```python
from build123d import *

# Parameters (mm, degrees)
SKETCH1_W           = 105
SKETCH1_H           = 100
BOSS_EXTRUDE1_DEPTH = 10
SKETCH4_R           = 15
BOSS_EXTRUDE2_DEPTH = 30
SKETCH5_R           = 4
CUT_EXTRUDE3_DEPTH  = 30
SKETCH6_W           = 42
SKETCH6_H           = 42
BOSS_EXTRUDE3_DEPTH = 1
SKETCH2_R           = 2.25
CUT_EXTRUDE4_DEPTH  = 99.994949366
BOSS_EXTRUDE4_START = 1
LOCAL_FILES1_R      = 6
LOCAL_FILES1_R_2    = 4
BOSS_EXTRUDE4_DEPTH = 1


with BuildPart() as part:
    # Sketch1 → Boss-Extrude1 (new body)
    with BuildSketch(Plane.XY):
        with Locations((-27.5, 0)):
            Rectangle(SKETCH1_W, SKETCH1_H)
    extrude(amount=BOSS_EXTRUDE1_DEPTH)

    # Sketch4 → Boss-Extrude2 (add)
    with BuildSketch(Plane.XY.offset(10)):
        Circle(SKETCH4_R)
    extrude(amount=BOSS_EXTRUDE2_DEPTH)

    # Sketch5 → Cut-Extrude3 (cut)
    with BuildSketch(Plane.XY.offset(40)):
        Circle(SKETCH5_R)
    extrude(amount=-CUT_EXTRUDE3_DEPTH, mode=Mode.SUBTRACT)

    # Sketch6 → Boss-Extrude3 (add)
    with BuildSketch(Plane.XY.offset(10)):
        with Locations((-59, 2.474517647)):
            Rectangle(SKETCH6_W, SKETCH6_H)
    extrude(amount=BOSS_EXTRUDE3_DEPTH)

    # Sketch2 → Cut-Extrude4 (cut, through all)
    with BuildSketch(Plane.XY.offset(10)):
        with Locations((-70, 40)):
            Circle(SKETCH2_R)
        with Locations((15, -40)):
            Circle(SKETCH2_R)
        with Locations(Location((-70, -40, 0), (0, 0, 180))):
            Circle(SKETCH2_R)
        with Locations(Location((15, 40, 0), (0, 0, 180))):
            Circle(SKETCH2_R)
    extrude(amount=-CUT_EXTRUDE4_DEPTH, mode=Mode.SUBTRACT)

    # Local Files1 → Boss-Extrude4 (add)
    with BuildSketch(Plane.XY.offset(40).offset(BOSS_EXTRUDE4_START)):
        Circle(LOCAL_FILES1_R)
        Circle(LOCAL_FILES1_R_2, mode=Mode.SUBTRACT)
    extrude(amount=-BOSS_EXTRUDE4_DEPTH)


solid = part.part
```
Here's how the part is built. I have some questions about the finished solid (model axes, mm). A direction names the side the tool comes from. Coordinates: 2 decimals unless noted, no trailing zeros. Order: outer loops, then holes, each group sorted by start corner. A loop starts at its lowest first (then second) coordinate and runs counter-clockwise, first axis right, second up. Notation, with made-up numbers: M 48.25,62 L 91.25,62 A17 cw 91.25,77 Z; hole C 39.5,-39 d3. An arc over 180 degrees is marked long. Answer as a JSON object with one key per item and string values. Group by question number.
(1) Suppose I cut it at A-A, the plane x = -65.5. Please give me the cut outline in (y, z).
(2) Suppose I cut it at C-C, the plane y = 40. Please give me the cut outline in (x, z), then the cut area to 3 significant figures.
(3) For pin 1 (0.8 mm diameter, centred on x = -53, z = 10.5, fed in from +Y); pin 2 (10 mm diameter, centred on x = 0, z = 24.5, fed in from -Y); pin 3 (1 mm diameter, centred on y = -10.5, z = 13, fed in from -X), each with a flat end and sliding along its axis, tell me the tip position at first contact or that it passes through.
(4) Suppose I cut it at B-B, the plane y = 0. Please give me the cut outline in (x, z), then the cut area to 3 significant figures.
(5) Which directions (+Z, -Z, +X, -X, +Y, -Y) give clear straight access to the entire face, cutting with the end or side of a thin tool? Please do faces 4 (the face through (-5.994, 0.264, 40.507)), 5 (the face through (-80, -1, 5)), 6 (the face through (-59, 3, 11)).
(6) If we mould it in two halves opening along X, with no side actions, what happens to faces 1 (the face through (25, -1, 5)), 2 (the face through (-1.42, -3.92, 41)), 3 (the face through (16.21, -38.103, 5.07))? For each: released by +X, released by -X, zero draft, split by the parting line, or undercut.
(7) Suppose I cut it at D-D, the plane z = 15.5. Please give me the cut outline in (x, y), then the cut area to 3 significant figures.
(8) I need wall thicknesses on probe 1 along Y at (x, z) = (-70, 4); probe 2 along Z at (x, y) = (-27, 20); probe 3 along Z at (x, y) = (3, 7). Which ranges of each line are inside material? Lowest first, please.
Values found:
{
 "1": {"outline": "M -50,0 L 50,0 L 50,10 L 23.47,10 L 23.47,11 L -18.53,11 L -18.53,10 L -50,10 Z"},
 "2": {"outline": "M -80,0 L -72.25,0 L -72.25,10 L -80,10 Z; M -67.75,0 L 12.75,0 L 12.75,10 L -67.75,10 Z; M 17.25,0 L 25,0 L 25,10 L 17.25,10 Z", "area": "960 mm^2"},
 "3": {"pin 1": "stops at y = 23.47", "pin 2": "stops at y = -15", "pin 3": "stops at x = -11.18"},
 "4": {"outline": "M -80,0 L 25,0 L 25,10 L 15,10 L 15,40 L 6,40 L 6,41 L 4,41 L 4,10 L -4,10 L -4,41 L -6,41 L -6,40 L -15,40 L -15,10 L -38,10 L -38,11 L -80,11 Z", "area": "1,760 mm^2"},
 "5": {"face 4": "+Z", "face 5": "+Z, -Z, -X, +Y, -Y", "face 6": "+Z, -X, +Y, -Y"},
 "6": {"face 1": "released by +X", "face 2": "zero draft", "face 3": "undercut"},
 "7": {"outline": "C 0,0 d30; hole C 0,0 d8", "area": "657 mm^2"},
 "8": {"probe 1": "y = -50 to -42.25, -37.75 to 37.75, 42.25 to 50", "probe 2": "z = 0 to 10", "probe 3": "z = 0 to 40"}
}
